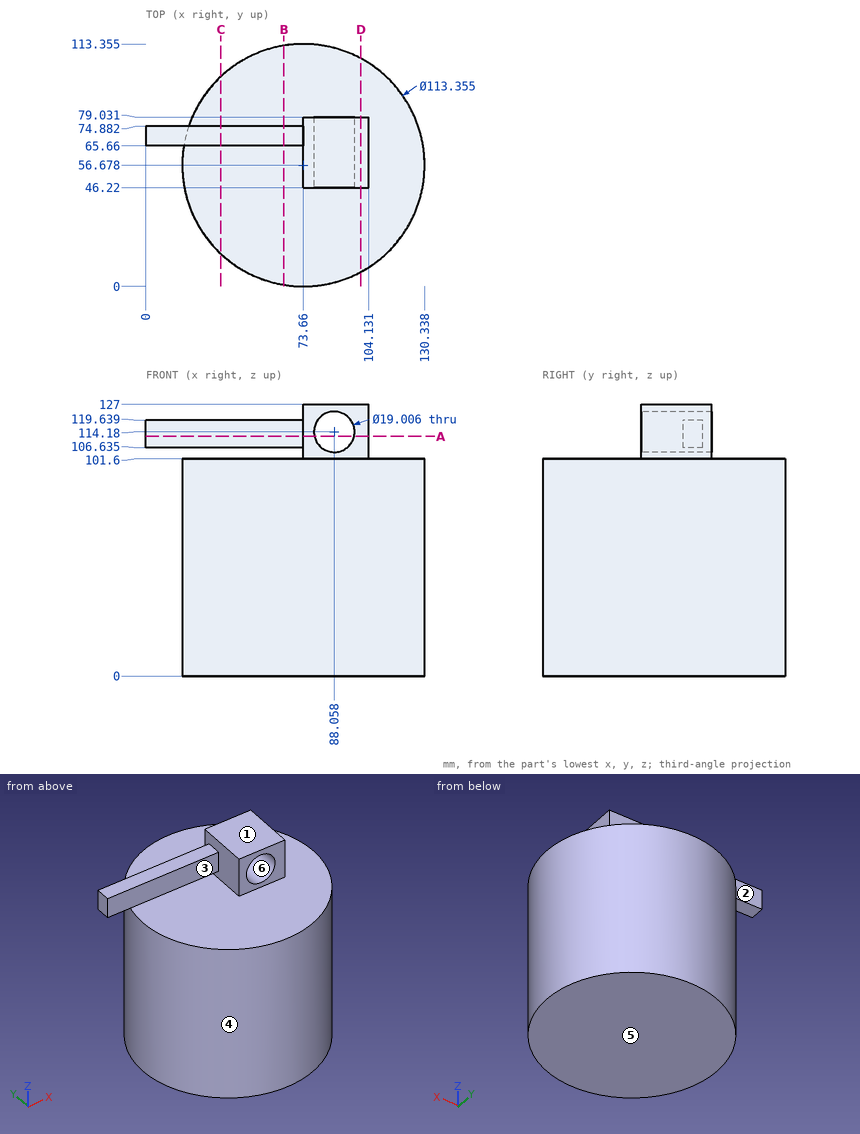
Input: dimensioned drawing with shaded views. Units: mm. Origin: part minimum x, y, z. A direction names the side the tool comes from. Give positions to 0.01 mm unless a question says otherwise; leave off trailing zeros. Write each loop counter-clockwise with the first axis right and the second up, starting at its lowest first coordinate (ties: lowest second). Pieces come first, ordered by that corner, then holes. Notation, with made-up numbers: (20.5, -2.5) -> (53.5, -2.5) arc R29 cw to (53.5, 26.5) -> close; hole circle Ø4 at (83.5, 28). An arc over 180 degrees is marked (long way). Return JSON: item names as keys, results as strings. Group by question number.
1. Access query for the marked faces 1, 2 and 3. Directions: +Z, -Z, +X, -X, +Y, -Y. A direction counts if a zero-diameter tool reaches every point of the face in a straight line with its end or side. Return the directions, or none.
2. Section C-C, the plane x = 35. Output: boundary loops of the cut face in (y, z) (1 decimal).
3. Section D-D, the plane x = 100.5. Output: boundary loops of the cut face in (y, z).
4. Section A-A, the plane z = 112. Output: boundary loops of the cut face in (x, y), then the cut area to 3 significant figures.
5. Section B-B, the plane x = 64.5. Output: boundary loops of the cut face in (y, z) (1 decimal).
6. Mould query, pull axis Z, two halves, no side actions, for the marked faces 4, 5 and 6. Classes: +Z half, -Z half, draft (parallel to the pull), parting line (faces both ways), or undercut.
7. Pin query (flat end, axial travel): pin 1 Ø4 at (y, z) = (44.5, 73) entering from +X; pin 2 Ø4 at (x, y) = (76, 97.5) entering from +Z; pin 3 Ø3 at (y, z) = (11.5, 58) entering from +X. Return the tip coordinate at first contact, or that it passes through.
8. Material intervals for line 1 (Z direction, x = 70, y = 73) (1 decimal); line 2 (Y direction, x = 21.5, z = 115.5); line 3 (X direction, y = 75, z = 111.5) (1 decimal), sorted ascending. Write a range as from..to.
Determined:
{
 "1": {"face 1": "+Z, +X, -X, +Y, -Y", "face 2": "+Z, -X, +Y", "face 3": "+Z, -X, -Y"},
 "2": {"outline": "(15.2, 0) -> (98.1, 0) -> (98.1, 101.6) -> (15.2, 101.6) -> close; (65.7, 106.6) -> (74.9, 106.6) -> (74.9, 119.6) -> (65.7, 119.6) -> close"},
 "3": {"outline": "(6.76, 0) -> (106.6, 0) -> (106.6, 101.6) -> (79.03, 101.6) -> (79.03, 127) -> (46.22, 127) -> (46.22, 101.6) -> (6.76, 101.6) -> close"},
 "4": {"outline": "(0, 65.66) -> (73.66, 65.66) -> (73.66, 46.22) -> (78.81, 46.22) -> (78.81, 79.03) -> (73.66, 79.03) -> (73.66, 74.88) -> (0, 74.88) -> close; (97.31, 46.22) -> (104.13, 46.22) -> (104.13, 79.03) -> (97.31, 79.03) -> close", "area": "1,070 mm2"},
 "5": {"outline": "(0.7, 0) -> (112.6, 0) -> (112.6, 101.6) -> (0.7, 101.6) -> close; (65.7, 106.6) -> (74.9, 106.6) -> (74.9, 119.6) -> (65.7, 119.6) -> close"},
 "6": {"face 4": "draft", "face 5": "-Z half", "face 6": "undercut"},
 "7": {"pin 1": "stops at x = 129.42", "pin 2": "stops at z = 101.6", "pin 3": "stops at x = 109.78"},
 "8": {"line 1": "z = 0..101.6, 106.6..119.6", "line 2": "y = 65.66..74.88", "line 3": "x = 73.7..78.9, 97.2..104.1"}
}
